```python
from build123d import *

# Parameters (mm, degrees)
SKETCH_1_W          = 44
SKETCH_1_H          = 44
SKETCH_1_W_2        = 40
SKETCH_1_H_2        = 40
EXTRUDE_1_DEPTH     = 20
SKETCH_2_W          = 44
SKETCH_2_H          = 44
EXTRUDE_1_2_DEPTH   = 2
SKETCH_3_R          = 2
CUT_EXTRUDE_1_DEPTH = 2


with BuildPart() as part:
    # 草图1 → Extrude 1 (new body)
    with BuildSketch(Plane(origin=(0, 0, 0), x_dir=(1, 0, 0), z_dir=(0, 1, 0))):
        Rectangle(SKETCH_1_W, SKETCH_1_H)
        Rectangle(SKETCH_1_W_2, SKETCH_1_H_2, mode=Mode.SUBTRACT)
    extrude(amount=EXTRUDE_1_DEPTH)

    # 草图2 → Extrude 1 2 (add)
    with BuildSketch(Plane(origin=(0, 20, 0), x_dir=(1, 0, 0), z_dir=(0, 1, 0))):
        Rectangle(SKETCH_2_W, SKETCH_2_H)
    extrude(amount=EXTRUDE_1_2_DEPTH)

    # 草图3 → 切除-拉伸1 (cut)
    with BuildSketch(Plane(origin=(0, 22, 0), x_dir=(1, 0, 0), z_dir=(0, 1, 0))):
        with Locations(Location((0, 0, 0), (0, 0, 270))):
            Circle(SKETCH_3_R)
    extrude(amount=-CUT_EXTRUDE_1_DEPTH, mode=Mode.SUBTRACT)


solid = part.part
```
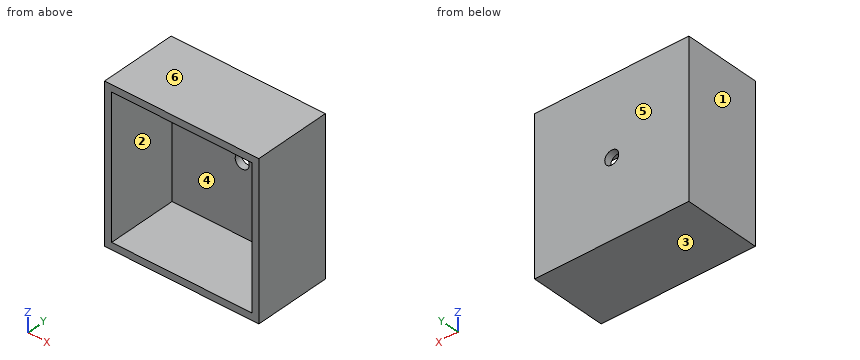
Part model, mm, in its own coordinate system. Face numbers are marked on the shaded views. A direction names the side the tool comes from. Round coordinates to 2 decimals unless told otherwise and drop trailing zeros. Loops run counter-clockwise (first coordinate to the right, second up) from the corner with the lowest first, then second, coordinate; pieces in that order, holes last. Notation, with made-up numbers: (46, -11) -> (88, -11) arc R28 ccw to (88, 10) -> close; hole circle Ø11 at (44.5, 79.25). An arc over 180 degrees is marked (long way). Use one line per item in the form item = value. Start each with the question number.
Item 1: Band-saw the part on B-B (z = 0). List the corners of the cut face in (x, y), plus the area to 3 significant figures.
Item 2: Band-saw the part on C-C (y = 16.75). List the corners of the cut face in (x, z), plus the area to 3 significant figures.
Item 3: Drill centre lines: line 1 along Z through (x, y) = (-10, 4); line 2 along X through (y, z) = (20.5, 0). Where is each one in solid material? Low to high.
Item 4: Drop a flat-ended pin along its axis: pin 1 Ø12 at (x, z) = (-3, 1) entering from -Y. Give the stop position or say it passes through.
Item 5: Tool access for the marked faces 1 and 2: list every direction of +Z, -Z, +X, -X, +Y, -Y with a clear straight run to the whole face (end or side of a thin tool).
Item 6: Band-saw the part on A-A (x = 0). List the corners of the cut face in (y, z).
Item 7: Two-plate mould, pull along Z, no slides. Class the marked faces 3, 4, 5 and 6: released by +Z, released by -Z, zero draft, split by the parting line, or undercut.
Item 8: Band-saw the part on D-D (z = -11). List the corners of the cut face in (x, y).
Data:
q1.outline = (-22, 0) -> (-20, 0) -> (-20, 20) -> (-2, 20) -> (-2, 22) -> (-22, 22) -> close; (2, 20) -> (20, 20) -> (20, 0) -> (22, 0) -> (22, 22) -> (2, 22) -> close
q1.area = 160 mm^2
q2.outline = (-22, -22) -> (22, -22) -> (22, 22) -> (-22, 22) -> close; hole (-20, -20) -> (20, -20) -> (20, 20) -> (-20, 20) -> close
q2.area = 336 mm^2
q3.line_1 = -22 to -20, 20 to 22
q3.line_2 = -22 to -2, 2 to 22
q4.pin_1 = 20
q5.face_1 = +Z, -Z, -X, +Y, -Y
q5.face_2 = -Y
q6.outline = (0, -22) -> (22, -22) -> (22, -2) -> (20, -2) -> (20, -20) -> (0, -20) -> close; (0, 20) -> (20, 20) -> (20, 2) -> (22, 2) -> (22, 22) -> (0, 22) -> close
q7.face_3 = released by -Z
q7.face_4 = undercut
q7.face_5 = zero draft
q7.face_6 = released by +Z
q8.outline = (-22, 0) -> (-20, 0) -> (-20, 20) -> (20, 20) -> (20, 0) -> (22, 0) -> (22, 22) -> (-22, 22) -> close
